from build123d import *

# Parameters (mm, degrees)
CROQUIS1_W              = 75
CROQUIS1_H              = 41
CROQUIS1_W_2            = 69
CROQUIS1_H_2            = 35
SALIENTE_EXTRUIR1_DEPTH = 22
CROQUIS1_2_W            = 69
CROQUIS1_2_H            = 35
SALIENTE_EXTRUIR2_DEPTH = 3
CROQUIS3_W              = 1.5
CROQUIS3_H              = 1.5
CORTAR_EXTRUIR1_DEPTH   = 72
CROQUIS4_W              = 38
CROQUIS4_H              = 1.5
CORTAR_EXTRUIR2_DEPTH   = 1.5
CROQUIS7_W              = 1.5
CROQUIS7_H              = 5
CORTAR_EXTRUIR3_DEPTH   = 0.3


with BuildPart() as part:
    # Croquis1 → Saliente-Extruir1 (new body)
    with BuildSketch(Plane(origin=(0, 0, 0), x_dir=(1, 0, 0), z_dir=(0, 1, 0))):
        Rectangle(CROQUIS1_W, CROQUIS1_H)
        Rectangle(CROQUIS1_W_2, CROQUIS1_H_2, mode=Mode.SUBTRACT)
    extrude(amount=SALIENTE_EXTRUIR1_DEPTH)

    # Croquis1_2 → Saliente-Extruir2 (add)
    with BuildSketch(Plane(origin=(0, 0, 0), x_dir=(1, 0, 0), z_dir=(0, 1, 0))):
        Rectangle(CROQUIS1_2_W, CROQUIS1_2_H)
    extrude(amount=SALIENTE_EXTRUIR2_DEPTH)

    # Croquis3 → Cortar-Extruir1 (cut)
    with BuildSketch(Plane.ZY.offset(37.5)):
        Polygon((17.5, 22), (-17.5, 22), (-17.5, 20.5), (-17.5, 19), (17.5, 19), (17.5, 20.5), align=None)
        with Locations((-18.25, 19.75)):
            Rectangle(CROQUIS3_W, CROQUIS3_H)
        with Locations((18.25, 19.75)):
            Rectangle(CROQUIS3_W, CROQUIS3_H)
    extrude(amount=-CORTAR_EXTRUIR1_DEPTH, mode=Mode.SUBTRACT)

    # Croquis4 → Cortar-Extruir2 (cut)
    with BuildSketch(Plane.ZY.offset(-34.5)):
        with Locations((0, 19.75)):
            Rectangle(CROQUIS4_W, CROQUIS4_H)
    extrude(amount=-CORTAR_EXTRUIR2_DEPTH, mode=Mode.SUBTRACT)

    # Croquis7 → Cortar-Extruir3 (cut)
    with BuildSketch(Plane(origin=(0, 19, 0), x_dir=(1, 0, 0), z_dir=(0, 1, 0))):
        with Locations((-36.121212609, 0)):
            Rectangle(CROQUIS7_W, CROQUIS7_H)
    extrude(amount=-CORTAR_EXTRUIR3_DEPTH, mode=Mode.SUBTRACT)


solid = part.part
The model under review builds one solid part; all positions refer to its coordinate system, in mm. A direction names the side the tool comes from. Coordinates: 2 decimals unless noted, no trailing zeros. Write each loop counter-clockwise with the first axis right and the second up, starting at its lowest first coordinate (ties: lowest second). Pieces come first, ordered by that corner, then holes. Notation, with made-up numbers: (20, 59.25) - (65, 59.25) arc R30 cw to (65, 98.25) - close; hole circle Ø10 at (72, 23.5). An arc over 180 degrees is marked (long way). Answer as a JSON object with one key per item and string values. Group by question number.
1. Clearance check with flat-ended pins moving along their axes: pin 1 Ø12 at (x, z) = (-6, -7.5) entering from +Y; pin 2 Ø1.2 at (y, z) = (20, -5.5) entering from -X. State where each tip first meets the part, or that it passes through.
2. Mouldability with a two-part tool opening along Y and no side actions: class faces 5 (the face through (-1, 20.5, 18)), 6 (the face through (-1, 20, 19)), 7 (the face through (-1, 0, 0)), 8 (the face through (-2, 21, 17.5)) as pulls with the +Y half, pulls with the -Y half, needs draft (parallel to the pull), parting line crosses it, or undercut.
3. Add section A-A (y = 13.25). Give the boundary of the cut face in (x, z).
4. Add section D-D (z = 10). Give the boundary of the cut face in (x, y).
5. Machinability: for faces 1 (the face through (-2, 21, -17.5)), 2 (the face through (-1, 11, 20.5)), 3 (the face through (0, 11, -17.5)), 4 (the face through (-1, 20, -19)), which of the approach directions +Z, -Z, +X, -X, +Y, -Y give a long, thin tool a straight path to every point of the face, cutting with its end or side? Answer none if there is none.
6. Add section B-B (x = 32). Give the boundary of the cut face in (y, z), plus the area to 4 significant figures.
7. Add section C-C (z = -1). Give the boundary of the cut face in (x, y).
8. To check wall thickness, follow probe 1 along X at (y, z) = (7, 6); probe 2 along Z at (x, y) = (-28, 5.25); probe 3 along Y at (x, z) = (18.5, -15.5). State the ranges of each line that lie inside material, in increasing order.
Findings:
{
 "1": {"pin 1": "y = 3", "pin 2": "x = 34.5"},
 "2": {"face 5": "undercut", "face 6": "undercut", "face 7": "pulls with the -Y half", "face 8": "needs draft"},
 "3": {"outline": "(-37.5, -20.5) - (37.5, -20.5) - (37.5, 20.5) - (-37.5, 20.5) - close; hole (-34.5, -17.5) - (34.5, -17.5) - (34.5, 17.5) - (-34.5, 17.5) - close"},
 "4": {"outline": "(-37.5, 0) - (37.5, 0) - (37.5, 22) - (34.5, 22) - (34.5, 20.5) - (36, 20.5) - (36, 19) - (34.5, 19) - (34.5, 3) - (-34.5, 3) - (-34.5, 19) - (-37.5, 19) - close"},
 "5": {"face 1": "-X, +Y", "face 2": "+Z, +X, -X, +Y, -Y", "face 3": "+Y", "face 4": "-X"},
 "6": {"outline": "(0, -20.5) - (22, -20.5) - (22, -17.5) - (20.5, -17.5) - (20.5, -19) - (19, -19) - (19, -17.5) - (3, -17.5) - (3, 17.5) - (19, 17.5) - (19, 19) - (20.5, 19) - (20.5, 17.5) - (22, 17.5) - (22, 20.5) - (0, 20.5) - close", "area": "232.5 mm²"},
 "7": {"outline": "(-37.5, 0) - (37.5, 0) - (37.5, 22) - (34.5, 22) - (34.5, 20.5) - (36, 20.5) - (36, 19) - (34.5, 19) - (34.5, 3) - (-34.5, 3) - (-34.5, 19) - (-35.37, 19) - (-35.37, 18.7) - (-36.87, 18.7) - (-36.87, 19) - (-37.5, 19) - close"},
 "8": {"probe 1": "-37.5 to -34.5, 34.5 to 37.5", "probe 2": "-20.5 to -17.5, 17.5 to 20.5", "probe 3": "0 to 3"}
}
